```python
from build123d import *

# Parameters (mm, degrees)
ESQUISSE1_R          = 1
BASE_EXTRUSION_DEPTH = 1.5


with BuildPart() as part:
    # Esquisse1 → Base-Extrusion (new body)
    with BuildSketch(Plane.XY):
        with BuildLine():
            Line((7.209029703, -9.507825682), (7.412373516, -9.776011223))
            ThreePointArc((7.412373516, -9.776011223), (7.597932232, -10.566966478), (7.135063159, -11.234644899))
            ThreePointArc((7.135063159, -11.234644899), (5.339769929, -12.152978871), (3.429352348, -12.798517198))
            Line((3.429352348, -12.798517198), (2.394076167, -8.934813893))
            ThreePointArc((2.394076167, -8.934813893), (0, 9.25), (-2.394076167, -8.934813893))
            Line((-2.394076167, -8.934813893), (-3.429352348, -12.798517198))
            ThreePointArc((-3.429352348, -12.798517198), (-5.339769929, -12.152978871), (-7.135063159, -11.234644899))
            ThreePointArc((-7.135063159, -11.234644899), (-7.597932232, -10.566966478), (-7.412373516, -9.776011223))
            Line((-7.412373516, -9.776011223), (-7.209029703, -9.507825682))
            ThreePointArc((-7.209029703, -9.507825682), (-7.011742469, -8.795467512), (-7.357625498, -8.142213086))
            ThreePointArc((-7.357625498, -8.142213086), (0, 11.85), (7.357625498, -8.142213086))
            ThreePointArc((7.357625498, -8.142213086), (7.011742469, -8.795467512), (7.209029703, -9.507825682))
        make_face()
        with Locations((4.764569663, -10.084729396)):
            Circle(ESQUISSE1_R, mode=Mode.SUBTRACT)
        with Locations(Location((-4.764569663, -10.084729396, 0), (0, 0, 180))):
            Circle(ESQUISSE1_R, mode=Mode.SUBTRACT)
    extrude(amount=BASE_EXTRUSION_DEPTH)


solid = part.part
```
The listing builds one solid part. Answer for the finished solid, in the listing's coordinates (mm). A direction names the side the tool comes from. Coordinates: 2 decimals unless noted, no trailing zeros. Write each loop counter-clockwise with the first axis right and the second up, starting at its lowest first coordinate (ties: lowest second). Pieces come first, ordered by that corner, then holes. Notation, with made-up numbers: (61, 38) - (76, 38) arc R16 cw to (76, 56) - close; hole circle Ø1 at (-26.5, 14.25). An arc over 180 degrees is marked (long way). Return JSON: item names as keys, results as strings. Group by question number.
1. A cutting plane is placed at B-B, the plane y = -10.5. Determine the outline of the cut face in (x, z), plus the area to 3 significant figures.
2. Determine the mould class of faces 1 (the cylindrical face through (-5.718, -10.385, 0.74)), 2 (the flat face through (2.92, -10.89, 0.74)), 3 (the flat face through (5, 8, 0)), 4 (the cylindrical face through (5.718, -9.784, 0.74)) for opening direction Y: released by +Y, released by -Y, zero draft, split by the parting line, or undercut.
3. A cutting plane is placed at A-A, the plane x = -5.25. Determine the outline of the cut face in (y, z).
4. A cutting plane is placed at C-C, the plane y = -3.5. Determine the outline of the cut face in (x, z).
5. Which of the six approach directions +Z, -Z, +X, -X, +Y, -Y give full straight-line access (tool end or side, diameter ignored) to faces 5 (the flat face through (-2.904, -10.84, 0.74)), 6 (the flat face through (5, 8, 1.5))?
6. Straight lines are drawn through the part: L1, parallel to Y at x = 7.5, z = 0.55; L2, parallel to Y at x = -4.5, z = 0.8; L3, parallel to X at y = -6, z = 1.2. For each, find the intervals that lie inside material, in ascending order.
7. A cutting plane is placed at D-D, the plane z = 1.25. Determine the outline of the cut face in (x, y).
Ans:
{
 "1": {"outline": "(-7.61, 0) - (-5.67, 0) - (-5.67, 1.5) - (-7.61, 1.5) - close; (-3.85, 0) - (-2.81, 0) - (-2.81, 1.5) - (-3.85, 1.5) - close; (2.81, 0) - (3.85, 0) - (3.85, 1.5) - (2.81, 1.5) - close; (5.67, 0) - (7.61, 0) - (7.61, 1.5) - (5.67, 1.5) - close", "area": "8.93 mm²"},
 "2": {"face 1": "undercut", "face 2": "released by -Y", "face 3": "zero draft", "face 4": "undercut"},
 "3": {"outline": "(-12.19, 0) - (-10.96, 0) - (-10.96, 1.5) - (-12.19, 1.5) - close; (-9.21, 0) - (-7.62, 0) - (-7.62, 1.5) - (-9.21, 1.5) - close; (7.62, 0) - (10.56, 0) - (10.56, 1.5) - (7.62, 1.5) - close"},
 "4": {"outline": "(-10.62, 0) - (-8.56, 0) - (-8.56, 1.5) - (-10.62, 1.5) - close; (8.56, 0) - (10.62, 0) - (10.62, 1.5) - (8.56, 1.5) - close"},
 "5": {"face 5": "+Z, -Z, -Y", "face 6": "+Z, +X, -X, +Y, -Y"},
 "6": {"L1": "-10.85 to -9.91, -8.02 to -5.41, 5.41 to 9.02", "L2": "-12.48 to -11.05, -9.12 to -8.08, 8.08 to 10.92", "L3": "-9.3 to -7.04, 7.04 to 9.3"},
 "7": {"outline": "(-7.41, -9.78) arc R1 ccw to (-7.14, -11.23) arc R13.73 ccw to (-3.43, -12.8) - (-2.39, -8.93) arc R9.25 cw (long way) to (2.39, -8.93) - (3.43, -12.8) arc R13.73 ccw to (7.14, -11.23) arc R1 ccw to (7.41, -9.78) - (7.21, -9.51) arc R1 cw to (7.36, -8.14) arc R11.35 ccw (long way) to (-7.36, -8.14) arc R1 cw to (-7.21, -9.51) - close; hole circle Ø2 at (-4.76, -10.08); hole circle Ø2 at (4.76, -10.08)"}
}
